Read the model definition and answer for the solid it produces. Units are mm, in the model's axes. Face numbers are marked on the shaded views. Coordinates: 2 decimals unless noted, no trailing zeros. Write each loop counter-clockwise with the first axis right and the second up, starting at its lowest first coordinate (ties: lowest second). Pieces come first, ordered by that corner, then holes. Notation, with made-up numbers: (-33, 35.25) -> (-27, 35.25) arc R14 cw to (-27, 46.25) -> close; hole circle Ø8 at (88.25, 52.25). An arc over 180 degrees is marked (long way). One line per item, written item: value. Start each with the question number.
1. Consider line 1 along X through (y, z) = (4.15, 0); line 2 along Y through (x, z) = (2.25, 12.5); line 3 along Y through (x, z) = (2.25, 1). Determine where each line is inside the solid, lowest interval first.
2. For a pull along X with two mould halves and no side action, classify the marked faces 1, 2 and 3 as pulls with the +X half, pulls with the -X half, needs draft (parallel to the pull), parting line crosses it, or undercut.
3. Given P1, Ø5, axis at x = 1.5, z = -0.5, coming from the +Y side; P2, Ø10, axis at x = 12.5, z = 9, coming from the -Y side; P3, Ø0.6, axis at x = -6.5, y = 1, coming from the +Z side; P4, Ø2, axis at y = 1.5, z = -6.5, coming from the +X side, each flat-ended and moving along its own axis, determine where each tip first touches the part or whether it passes through.
4. Find section A-A, the plane y = 2.5. Write down the section's boundary in (x, z).
5. Find section B-B, the plane x = 13.5. Write down the section's boundary in (y, z).
```python
from build123d import *

# Parameters (mm, degrees)
SKETCH_1_R          = 9
SKETCH_1_R_2        = 7.5
EXTRUDE_1_DEPTH     = 6
EXTRUDE_START       = -1
EXTRUDE_2_DEPTH     = 1
EXTRUDE_3_DEPTH     = 3
EXTRUDE_START_2     = -3
SKETCH_5_R          = 7.5
EXTRUDE_4_DEPTH     = 3
SKETCH_6_R          = 1.6
CUT_EXTRUDE_1_DEPTH = 3
SKETCH_7_R          = 3
CUT_EXTRUDE_2_DEPTH = 1.5
CHAMFER_1_SIZE      = 1


with BuildPart() as part:
    # 草图1 → 凸台-拉伸1 (new body)
    with BuildSketch(Plane(origin=(0, 0, 0), x_dir=(1, 0, 0), z_dir=(0, 1, 0))):
        with Locations(Location((0, 0, 0), (0, 0, 270))):
            Circle(SKETCH_1_R)
        with Locations(Location((0, 0, 0), (0, 0, 270))):
            Circle(SKETCH_1_R_2, mode=Mode.SUBTRACT)
    extrude(amount=EXTRUDE_1_DEPTH)

    # 草图2 → 凸台-拉伸2 (add)
    with BuildSketch(Plane(origin=(0, 6, 0), x_dir=(1, 0, 0), z_dir=(0, 1, 0)).offset(EXTRUDE_START)):
        with BuildLine():
            Line((0, 20), (0, 9))
            ThreePointArc((0, 9), (6.363961031, 6.363961031), (9, 0))
            ThreePointArc((9, 0), (6.363961031, -6.363961031), (0, -9))
            Line((0, -9), (0, -20))
            ThreePointArc((0, -20), (14.142135624, -14.142135624), (20, 0))
            ThreePointArc((20, 0), (14.142135624, 14.142135624), (0, 20))
        make_face()
    extrude(amount=EXTRUDE_2_DEPTH)

    # 草图4 → 凸台-拉伸3 (add)
    with BuildSketch(Plane.XZ):
        with BuildLine():
            Line((0.856553191, 6.326082651), (0.856553191, 7.450927233))
            ThreePointArc((0.856553191, 7.450927233), (-0.043739259, 7.499872457), (-0.943399591, 7.440429908))
            Line((-0.943399591, 7.440429908), (-0.943399591, 6.312339741))
            Line((-0.943399591, 6.312339741), (-0.943399591, 5.418486616))
            ThreePointArc((-0.943399591, 5.418486616), (-0.044016518, 5.499823865), (0.856553191, 5.432892106))
            Line((0.856553191, 5.432892106), (0.856553191, 6.326082651))
        make_face()
        with BuildLine():
            Line((6.312339741, 0.943399591), (5.418486616, 0.943399591))
            ThreePointArc((5.418486616, 0.943399591), (5.499823865, 0.044016518), (5.432892106, -0.856553191))
            Line((5.432892106, -0.856553191), (6.326082651, -0.856553191))
            Line((6.326082651, -0.856553191), (7.450927233, -0.856553191))
            ThreePointArc((7.450927233, -0.856553191), (7.499872457, 0.043739259), (7.440429908, 0.943399591))
            Line((7.440429908, 0.943399591), (6.312339741, 0.943399591))
        make_face()
        with BuildLine():
            Line((0.943399591, -6.312339741), (0.943399591, -5.418486616))
            ThreePointArc((0.943399591, -5.418486616), (0.044016518, -5.499823865), (-0.856553191, -5.432892106))
            Line((-0.856553191, -5.432892106), (-0.856553191, -6.326082651))
            Line((-0.856553191, -6.326082651), (-0.856553191, -7.450927233))
            ThreePointArc((-0.856553191, -7.450927233), (0.043739259, -7.499872457), (0.943399591, -7.440429908))
            Line((0.943399591, -7.440429908), (0.943399591, -6.312339741))
        make_face()
        with BuildLine():
            Line((-6.312339741, -0.943399591), (-5.418486616, -0.943399591))
            ThreePointArc((-5.418486616, -0.943399591), (-5.499823865, -0.044016518), (-5.432892106, 0.856553191))
            Line((-5.432892106, 0.856553191), (-6.326082651, 0.856553191))
            Line((-6.326082651, 0.856553191), (-7.450927233, 0.856553191))
            ThreePointArc((-7.450927233, 0.856553191), (-7.499872457, -0.043739259), (-7.440429908, -0.943399591))
            Line((-7.440429908, -0.943399591), (-6.312339741, -0.943399591))
        make_face()
    extrude(amount=-EXTRUDE_3_DEPTH)

    # 草图5 → 凸台-拉伸4 (add)
    with BuildSketch(Plane(origin=(0, 6, 0), x_dir=(1, 0, 0), z_dir=(0, 1, 0)).offset(EXTRUDE_START_2)):
        Circle(SKETCH_5_R)
    extrude(amount=EXTRUDE_4_DEPTH)

    # 草图6 → 切除-拉伸1 (cut)
    with BuildSketch(Plane(origin=(0, 6, 0), x_dir=(1, 0, 0), z_dir=(0, 1, 0))):
        with Locations(Location((0, 0, 0), (0, 0, 270))):
            Circle(SKETCH_6_R)
    extrude(amount=-CUT_EXTRUDE_1_DEPTH, mode=Mode.SUBTRACT)

    # 草图7 → 切除-拉伸2 (cut)
    with BuildSketch(Plane(origin=(0, 6, 0), x_dir=(1, 0, 0), z_dir=(0, 1, 0))):
        with Locations(Location((0, 0, 0), (0, 0, 270))):
            Circle(SKETCH_7_R)
    extrude(amount=-CUT_EXTRUDE_2_DEPTH, mode=Mode.SUBTRACT)

    # 倒角1
    chamfer_1_edges = [part.edges().sort_by_distance(p)[0] for p in [
        (0, 0, -9),
    ]]
    chamfer(chamfer_1_edges, length=CHAMFER_1_SIZE)


solid = part.part
```
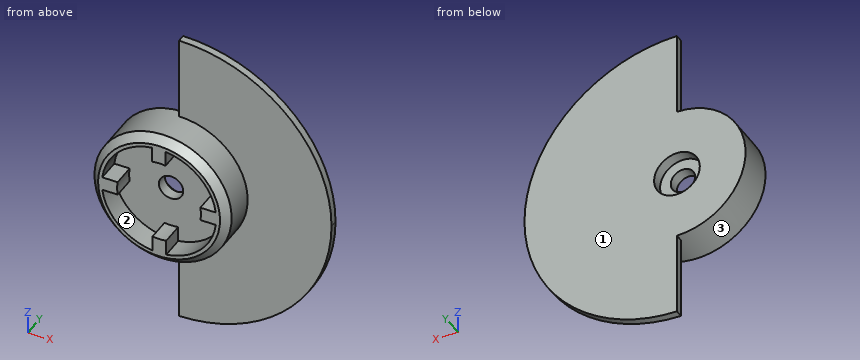
Answer block:
1. line 1: x = -9 to -1.6, 1.6 to 9
1. line 2: y = 5 to 6
1. line 3: y = 3 to 4.5
2. face 1: needs draft
2. face 2: undercut
2. face 3: parting line crosses it
3. P1: stops at y = 6
3. P2: stops at y = 5
3. P3: stops at z = 6.52
3. P4: stops at x = 7.12
4. outline: circle Ø18 at (0, 0); hole (-7.45, 0.86) -> (-5.43, 0.86) arc R5.5 ccw to (-5.42, -0.94) -> (-7.44, -0.94) arc R7.5 ccw to (-0.86, -7.45) -> (-0.86, -5.43) arc R5.5 ccw to (0.94, -5.42) -> (0.94, -7.44) arc R7.5 ccw to (7.45, -0.86) -> (5.43, -0.86) arc R5.5 ccw to (5.42, 0.94) -> (7.44, 0.94) arc R7.5 ccw to (0.86, 7.45) -> (0.86, 5.43) arc R5.5 ccw to (-0.94, 5.42) -> (-0.94, 7.44) arc R7.5 ccw to start
5. outline: (5, -14.76) -> (6, -14.76) -> (6, 14.76) -> (5, 14.76) -> close
